Build history of the part. All positions in model axes, mm. A direction names the side the tool comes from. Give positions to 0.01 mm unless a question says otherwise; leave off trailing zeros. Write each loop counter-clockwise with the first axis right and the second up, starting at its lowest first coordinate (ties: lowest second). Pieces come first, ordered by that corner, then holes. Notation, with made-up numbers: (34.25, 56) -> (50.25, 56) arc R27 ccw to (50.25, 75) -> close; hole circle Ø8 at (-14, -33.5). An arc over 180 degrees is marked (long way). One line per question, with ' | ' between items. Start each with the question number.
(1) Band-saw the part on A-A, the plane y = 0. Give the cut face in (x, z).
(2) Tool access for faces 3 (the flat face through (-11.5, -34, 50)), 4 (the flat face through (14.715, 25.16, 32.045)): list every direction of +Z, -Z, +X, -X, +Y, -Y with a clear straight run to the whole face (end or side of a thin tool).
(3) Pin check, flat tips, straight feed: P1, Ø2, axis at y = -33, z = 45.5, coming from the +X side; P2, Ø1, axis at y = -17, z = 33, coming from the +X side; P3, Ø7.5, axis at x = 29, z = 38, coming from the -Y side. Stop position of each tip, or through.
(4) Drill centre lines: probe 1 along X at (y, z) = (0, 57); probe 2 along Y at (x, z) = (-1, 60); probe 3 along Y at (x, z) = (0, 3). Where is each one in solid material? Low to high. Write a range as from..to.
(5) Band-saw the part on D-D, the plane y = -27. Give the cut face in (x, z), and give its area (3 significant figures).
(6) Band-saw the part on B-B, the plane x = 0. Give the cut face in (y, z), and give its area (3 significant figures).
(7) Band-saw the part on C-C, the plane z = 60. Count the separate pieces of the cut face and the enclosed holes in it, and give its area (3 significant figures).
(8) Pull direction Y, two halves, no side cores. Call faces 1 (the flat face through (28.11, -7.7, 32.04)), 2 (the flat face through (15.374, -18.429, 32.045)): released by +Y, released by -Y, zero draft, split by the parting line, or undercut.
from build123d import *

# Parameters (mm, degrees)
SKETCH2_R                       = 4.79
BOSS_EXTRUDE2_DEPTH             = 65
SHELL4_START                    = 5
SHELL4_OUTLINE_R                = 4.79
SHELL4_DEPTH                    = 60
SKETCH3_W                       = 42
SKETCH3_H                       = 12
BOSS_EXTRUDE3_DEPTH             = 65
SKETCH4_W                       = 23
SKETCH4_H                       = 4
CUT_EXTRUDE1_DEPTH              = 30
BOSS_EXTRUDE4_DEPTH             = 60
CIRPATTERN2_COUNT               = 3
CIRPATTERN2_ANGLE               = 50
CIRPATTERN2_THE_OTHER_WAY_COUNT = 3
CIRPATTERN2_THE_OTHER_WAY_ANGLE = 50
CUT_EXTRUDE2_START              = -5
SKETCH5_4_W                     = 9.6
SKETCH5_4_H                     = 9.8
CUT_EXTRUDE2_DEPTH              = 65
CIRPATTERN3_COUNT               = 3
CIRPATTERN3_ANGLE               = 50
CIRPATTERN3_THE_OTHER_WAY_COUNT = 3
CIRPATTERN3_THE_OTHER_WAY_ANGLE = 50
MIRROR1_OUTLINE_W               = 9.6
MIRROR1_OUTLINE_H               = 9.8
MIRROR1_DEPTH                   = 65
MIRROR1_START                   = 5
MIRROR1_2_DEPTH                 = 60
FILLET1_R                       = 8


# Read off the part's stored shape, not the designer's step: Shell4, Mirror1
with BuildPart() as part:
    # Sketch2 → Boss-Extrude2 (new body)
    with BuildSketch(Plane.XY):
        with BuildLine():
            Line((18.027756377, 30), (-18.027756377, 30))
            ThreePointArc((-18.027756377, 30), (-34.954133403, 1.791244829), (-21, -28))
            Line((-21, -28), (21, -28))
            ThreePointArc((21, -28), (34.954133403, 1.791244829), (18.027756377, 30))
        make_face()
        Circle(SKETCH2_R, mode=Mode.SUBTRACT)
    extrude(amount=BOSS_EXTRUDE2_DEPTH)

    # Shell4 outline → Shell4 (cut)
    with BuildSketch(Plane.XY.offset(SHELL4_START)):
        with BuildLine():
            ThreePointArc((-17.464249197, 28), (-32.953872935, 1.744207141), (-20.322401433, -26))
            Line((-20.322401433, -26), (20.322401433, -26))
            ThreePointArc((20.322401433, -26), (32.953872935, 1.744207141), (17.464249197, 28))
            Line((17.464249197, 28), (-17.464249197, 28))
        make_face()
        Circle(SHELL4_OUTLINE_R, mode=Mode.SUBTRACT)
    extrude(amount=SHELL4_DEPTH, mode=Mode.SUBTRACT)

    # Sketch3 → Boss-Extrude3 (add)
    with BuildSketch(Plane.XY.offset(65)):
        with Locations((0, -34)):
            Rectangle(SKETCH3_W, SKETCH3_H)
    extrude(amount=-BOSS_EXTRUDE3_DEPTH)

    # Sketch4 → Cut-Extrude1 (cut)
    with BuildSketch(Plane.XY.offset(65)):
        with Locations((0, -34)):
            Rectangle(SKETCH4_W, SKETCH4_H)
    extrude(amount=-CUT_EXTRUDE1_DEPTH, mode=Mode.SUBTRACT)

    # Sketch5 → Boss-Extrude4 (add)
    with BuildSketch(Plane.XY.offset(5)):
        with BuildLine():
            Line((24, 0), (23.2, 0))
            Line((23.2, 0), (23.2, -6))
            Line((23.2, -6), (32.136427928, -7.5))
            ThreePointArc((32.136427928, -7.5), (32.411387807, -6.204993184), (32.634184531, -4.9))
            Line((32.634184531, -4.9), (24, -4.9))
            Line((24, -4.9), (24, 0))
        make_face()
        with BuildLine():
            Line((23.2, 6), (23.2, 0))
            Line((23.2, 0), (24, 0))
            Line((24, 0), (24, 4.9))
            Line((24, 4.9), (32.634184531, 4.9))
            ThreePointArc((32.634184531, 4.9), (32.411387807, 6.204993184), (32.136427928, 7.5))
            Line((32.136427928, 7.5), (23.2, 6))
        make_face()
        with BuildLine():
            Line((33, 0), (24, 0))
            Line((24, 0), (24, -4.9))
            Line((24, -4.9), (32.634184531, -4.9))
            ThreePointArc((32.634184531, -4.9), (32.908419056, -2.456818113), (33, 0))
        make_face()
        with BuildLine():
            Line((24, 4.9), (24, 0))
            Line((24, 0), (33, 0))
            ThreePointArc((33, 0), (32.908419056, 2.456818113), (32.634184531, 4.9))
            Line((32.634184531, 4.9), (24, 4.9))
        make_face()
    boss_extrude4 = extrude(amount=BOSS_EXTRUDE4_DEPTH)

    # CirPattern2: Boss-Extrude4 ×3 about axis
    cirpattern2_axis = Axis((0, 0, 0), (0, 0, -1))
    for i in range(1, CIRPATTERN2_COUNT):
        add(boss_extrude4.rotate(cirpattern2_axis, i * CIRPATTERN2_ANGLE / (CIRPATTERN2_COUNT - 1)))

    # CirPattern2 the other way: Boss-Extrude4 ×3 about axis
    cirpattern2_the_other_way_axis = Axis((0, 0, 0), (0, 0, 1))
    for i in range(1, CIRPATTERN2_THE_OTHER_WAY_COUNT):
        add(boss_extrude4.rotate(cirpattern2_the_other_way_axis, i * CIRPATTERN2_THE_OTHER_WAY_ANGLE / (CIRPATTERN2_THE_OTHER_WAY_COUNT - 1)))

    # Sketch5<4> → Cut-Extrude2 (cut)
    with BuildSketch(Plane.XY.offset(5).offset(CUT_EXTRUDE2_START)):
        with Locations((28.8, 0)):
            Rectangle(SKETCH5_4_W, SKETCH5_4_H)
    cut_extrude2 = extrude(amount=CUT_EXTRUDE2_DEPTH, mode=Mode.SUBTRACT)

    # CirPattern3: Cut-Extrude2 ×3 about axis
    cirpattern3_axis = Axis((0, 0, 0), (0, 0, 1))
    for i in range(1, CIRPATTERN3_COUNT):
        add(cut_extrude2.rotate(cirpattern3_axis, i * CIRPATTERN3_ANGLE / (CIRPATTERN3_COUNT - 1)), mode=Mode.SUBTRACT)

    # CirPattern3 the other way: Cut-Extrude2 ×3 about axis
    cirpattern3_the_other_way_axis = Axis((0, 0, 0), (0, 0, -1))
    for i in range(1, CIRPATTERN3_THE_OTHER_WAY_COUNT):
        add(cut_extrude2.rotate(cirpattern3_the_other_way_axis, i * CIRPATTERN3_THE_OTHER_WAY_ANGLE / (CIRPATTERN3_THE_OTHER_WAY_COUNT - 1)), mode=Mode.SUBTRACT)

    # Mirror1 outline → Mirror1 (cut)
    with BuildSketch(Plane.XY):
        with Locations((-28.8, 0)):
            Rectangle(MIRROR1_OUTLINE_W, MIRROR1_OUTLINE_H)
        Polygon((-19.680557406, 14.583746438), (-28.381112162, 18.640881751), (-32.522771127, 9.759065438), (-23.822216371, 5.701930125), align=None)
        Polygon((-28.381112162, -18.640881751), (-19.680557406, -14.583746438), (-23.822216371, -5.701930125), (-32.522771127, -9.759065438), align=None)
        Polygon((-11.673284861, 21.534725922), (-17.844045914, 28.888752576), (-25.351281457, 22.589434001), (-19.180520404, 15.235407347), align=None)
        Polygon((-17.844045914, -28.888752576), (-11.673284861, -21.534725922), (-19.180520404, -15.235407347), (-25.351281457, -22.589434001), align=None)
    extrude(amount=MIRROR1_DEPTH, mode=Mode.SUBTRACT)

    # Mirror1 2 outline → Mirror1 2 (add)
    with BuildSketch(Plane.XY.offset(MIRROR1_START)):
        with BuildLine():
            ThreePointArc((-31.647445046, 9.350894183), (-32.217768235, 7.14250726), (-32.63418453, 4.9))
            Line((-32.63418453, 4.9), (-24, 4.9))
            Line((-24, 4.9), (-24, -4.9))
            Line((-24, -4.9), (-32.63418453, -4.9))
            ThreePointArc((-32.63418453, -4.9), (-32.217768234, -7.14250726), (-31.647445046, -9.350894183))
            Line((-31.647445046, -9.350894183), (-23.822216371, -5.701930125))
            Line((-23.822216371, -5.701930125), (-19.680557406, -14.583746438))
            Line((-19.680557406, -14.583746438), (-27.505786081, -18.232710496))
            ThreePointArc((-27.505786081, -18.232710496), (-26.18066023, -20.089127157), (-24.73046724, -21.849576428))
            Line((-24.73046724, -21.849576428), (-19.180520404, -15.235407347))
            Line((-19.180520404, -15.235407347), (-11.673284861, -21.534725922))
            Line((-11.673284861, -21.534725922), (-15.420094693, -26))
            Line((-15.420094693, -26), (-12.888229067, -26))
            Line((-12.888229067, -26), (-10.316405886, -21.628956738))
            Line((-10.316405886, -21.628956738), (-18.852681319, -14.466171171))
            Line((-18.852681319, -14.466171171), (-23.2, -5.143316173))
            Line((-23.2, -5.143316173), (-23.2, 5.143316173))
            Line((-23.2, 5.143316173), (-18.852681319, 14.466171171))
            Line((-18.852681319, 14.466171171), (-10.316405886, 21.628956738))
            Line((-10.316405886, 21.628956738), (-14.064983918, 28))
            Line((-14.064983918, 28), (-17.098293955, 28))
            Line((-17.098293955, 28), (-11.673284861, 21.534725922))
            Line((-11.673284861, 21.534725922), (-19.180520404, 15.235407347))
            Line((-19.180520404, 15.235407347), (-24.73046724, 21.849576428))
            ThreePointArc((-24.73046724, 21.849576428), (-26.18066023, 20.089127157), (-27.505786081, 18.232710496))
            Line((-27.505786081, 18.232710496), (-19.680557406, 14.583746438))
            Line((-19.680557406, 14.583746438), (-23.822216371, 5.701930125))
            Line((-23.822216371, 5.701930125), (-31.647445046, 9.350894183))
        make_face()
    extrude(amount=MIRROR1_2_DEPTH)

    # Fillet1
    # the kernel refuses this fillet: 8 mm, written as the material it adds along each edge
    with BuildSketch(Plane(origin=(14.064983918, 28, 5), x_dir=(-0.507111132951345, -0.8618806755211555, 0), z_dir=(0, 0, 1))) as fillet1_piece_1:
        with BuildLine():
            CenterArc((12.767888624, -5.924532666), FILLET1_R, 132.220297842, 78.251296778)
            Line((5.87284322, -9.98142173), (5.734942312, -10.062559511))
            Line((5.734942312, -10.062559511), (-0.137900908, -0.081137781))
            Line((-0.137900908, -0.081137781), (0, 0.16))
            ThreePointArc((0, 0.16), (3.696012361, 0.16), (7.284507445, 0.118490653))
            Line((7.284507445, 0.118490653), (7.392024723, 0))
        make_face()
    extrude(amount=60)
    with BuildSketch(Plane(origin=(-12.888229067, -26, 5), x_dir=(0.5071111329155005, 0.8618806755422457, 0), z_dir=(0, 0, 1))) as fillet1_piece_2:
        with BuildLine():
            CenterArc((11.814726499, -4.304548479), FILLET1_R, 147.447746104, 63.023848513)
            Line((4.919681094, -8.361437543), (4.781780186, -8.442575324))
            Line((4.781780186, -8.442575324), (-0.137900908, -0.081137781))
            Line((-0.137900908, -0.081137781), (0, 0.16))
            ThreePointArc((0, 0.16), (2.535758943, 0.16), (4.936653714, 0.08609097))
            Line((4.936653714, 0.08609097), (5.071517886, 0))
        make_face()
    extrude(amount=60)
    with BuildSketch(Plane(origin=(-14.064983918, 28, 5), x_dir=(1, 0, 0), z_dir=(0, 0, 1))) as fillet1_piece_3:
        with BuildLine():
            CenterArc((11.580978682, -8), FILLET1_R, 90, 78.251296781)
            Line((3.748578032, -6.371043262), (3.591930019, -6.338464127))
            ThreePointArc((3.591930019, -6.338464127), (1.736388108, -3.266659412), (-0.137900908, -0.081137781))
            Line((-0.137900908, -0.081137781), (0, 0.16))
            Line((0, 0.16), (11.580978682, 0.16))
            Line((11.580978682, 0.16), (11.580978682, 0))
        make_face()
    extrude(amount=60)
    with BuildSketch(Plane(origin=(12.888229067, -26, 65), x_dir=(-1, 0, 0), z_dir=(0, 0, -1))) as fillet1_piece_4:
        with BuildLine():
            CenterArc((9.701386491, 8), FILLET1_R, 206.97615149, 63.02384851)
            Line((2.571823181, 4.371043262), (2.429231915, 4.298464127))
            ThreePointArc((2.429231915, 4.298464127), (1.148010682, 2.266659412), (-0.137900908, 0.081137781))
            Line((-0.137900908, 0.081137781), (0, -0.16))
            Line((0, -0.16), (9.701386491, -0.16))
            Line((9.701386491, -0.16), (9.701386491, 0))
        make_face()
    extrude(amount=60)


solid = part.part
Results:
1) outline: (-35, 0) -> (-33.6, 0) -> (-33.6, 65) -> (-35, 65) -> close; (-24, 0) -> (-4.79, 0) -> (-4.79, 5) -> (-23.2, 5) -> (-23.2, 65) -> (-24, 65) -> close; (4.79, 0) -> (24, 0) -> (24, 65) -> (23.2, 65) -> (23.2, 5) -> (4.79, 5) -> close; (33.6, 0) -> (35, 0) -> (35, 65) -> (33.6, 65) -> close
2) face 3: +Z | face 4: +Z, -Z
3) P1: stops at x = 21 | P2: stops at x = 30.87 | P3: stops at y = -24.24
4) probe 1: x = -35..-33.6, -24..-23.2, 23.2..24, 33.6..35 | probe 2: y = -40..-36, -32..-26, 28..30 | probe 3: y = -40..-4.79, 4.79..30
5) outline: (-22.27, 0) -> (-20.09, 0) -> (-20.09, 65) -> (-22.27, 65) -> close; (-16.26, 0) -> (16.26, 0) -> (16.26, 65) -> (-16.26, 65) -> close; (20.09, 0) -> (22.27, 0) -> (22.27, 65) -> (20.09, 65) -> close | area: 2,400 mm²
6) outline: (-40, 0) -> (-4.79, 0) -> (-4.79, 5) -> (-26, 5) -> (-26, 65) -> (-32, 65) -> (-32, 35) -> (-36, 35) -> (-36, 65) -> (-40, 65) -> close; (4.79, 0) -> (30, 0) -> (30, 65) -> (28, 65) -> (28, 5) -> (4.79, 5) -> close | area: 1,140 mm²
7) separate pieces: 1 | enclosed holes: 12 | area: 1,140 mm²
8) face 1: undercut | face 2: undercut
